```python
from build123d import *

# Parameters (mm, degrees)
SKETCH6_R           = 26
BOSS_EXTRUDE1_DEPTH = 10
CUT_EXTRUDE3_DEPTH  = 39.105117767
CIRPATTERN2_COUNT   = 24
CUT_EXTRUDE4_DEPTH  = 38.897178127
SKETCH9_R           = 5
BOSS_EXTRUDE2_DEPTH = 4


with BuildPart() as part:
    # Sketch6 → Boss-Extrude1 (new body)
    with BuildSketch(Plane.XY):
        Circle(SKETCH6_R)
    extrude(amount=BOSS_EXTRUDE1_DEPTH)

    # Sketch7 → Cut-Extrude3 (cut, through all)
    with BuildSketch(Plane.XY.offset(10)):
        with BuildLine():
            ThreePointArc((-0.990237597, 21.477183929), (-1.515765167, 23.822734617), (-2.811039843, 25.847592828))
            ThreePointArc((-2.811039843, 25.847592828), (0, 26), (2.811039843, 25.847592828))
            ThreePointArc((2.811039843, 25.847592828), (1.515765167, 23.822734617), (0.990237597, 21.477183929))
            ThreePointArc((0.990237597, 21.477183929), (0, 21.5), (-0.990237597, 21.477183929))
        make_face()
    cut_extrude3 = extrude(amount=-CUT_EXTRUDE3_DEPTH, mode=Mode.SUBTRACT)

    # CirPattern2: Cut-Extrude3 ×24 about axis
    cirpattern2_axis = Axis((0, 0, 0), (0, 0, 1))
    for i in range(1, CIRPATTERN2_COUNT):
        add(cut_extrude3.rotate(cirpattern2_axis, i * 360 / CIRPATTERN2_COUNT), mode=Mode.SUBTRACT)

    # Sketch8 → Cut-Extrude4 (cut, through all)
    with BuildSketch(Plane.XY.offset(10)):
        with BuildLine():
            Line((-1.658312395, 2.5), (1.658312395, 2.5))
            ThreePointArc((1.658312395, 2.5), (0, -3), (-1.658312395, 2.5))
        make_face()
    extrude(amount=-CUT_EXTRUDE4_DEPTH, mode=Mode.SUBTRACT)

    # Sketch9 → Boss-Extrude2 (add)
    with BuildSketch(Plane(origin=(0, 0, 0), x_dir=(-1, 0, 0), z_dir=(0, 0, -1))):
        with Locations(Location((0, 0, 0), (0, 0, 180))):
            Circle(SKETCH9_R)
        with BuildLine():
            Line((-1.658312395, 2.5), (1.658312395, 2.5))
            ThreePointArc((1.658312395, 2.5), (0, -3), (-1.658312395, 2.5))
        make_face(mode=Mode.SUBTRACT)
    extrude(amount=BOSS_EXTRUDE2_DEPTH)


solid = part.part
```
Build history of the part. All positions in model axes, mm. A direction names the side the tool comes from. Round coordinates to 2 decimals unless told otherwise and drop trailing zeros. Write each loop counter-clockwise with the first axis right and the second up, starting at its lowest first coordinate (ties: lowest second). Pieces come first, ordered by that corner, then holes.
1) Band-saw the part on B-B, the plane y = -2. List the corners of the cut face in (x, z).
2) Pin check, flat tips, straight feed: pin 1 (2 mm diameter, centred on x = 7, z = 6, fed in from +Y); pin 2 (1 mm diameter, centred on x = -1, z = -1.5, fed in from -Y); pin 3 (2.5 mm diameter, centred on x = 0.5, z = 6.5, fed in from -Y). Stop position of each tip, or through.
3) 3-axis set-ups, long thin cutter, end or side, ignore diameter. For faces 1 (the cylindrical face through (-23.791, -1.503, 5.07)), 2 (the cylindrical face through (22.645, -7.651, 5.07)), 3 (the cylindrical face through (-23.37, 4.706, 5.07)): which of +Z, -Z, +X, -X, +Y, -Y reach the whole face in a straight line?
4) Band-saw the part on D-D, the plane z = -2.5. List the corners of the cut face in (x, y).
5) Drill centre lines: probe 1 along X at (y, z) = (-22, 5.75); probe 2 along X at (y, z) = (20, 8); probe 3 along Y at (x, z) = (0, -1.05). Where is each one in solid material? Low to high.
6) Band-saw the part on C-C, the plane x = 23. List the corners of the cut face in (y, z), and give its area (3 significant figures).
7) Band-saw the part on A-A, the plane x = 0. List the corners of the cut face in (y, z), and give its area (3 significant figures).
8) Mould opens along X. For faces 4 (the cylindrical face through (10.738, -18.626, 5.07)), 5 (the cylindrical face through (-22.59, -7.61, 5.07)), 6 (the cylindrical face through (25.776, -3.402, 4.93)) say: +X half, -X half, draft (parallel to the pull), parting line (faces both ways), or undercut.
Ans:
1. outline: (-24.77, 0) - (-4.58, 0) - (-4.58, -4) - (-2.24, -4) - (-2.24, 10) - (-24.77, 10) - close; (2.24, -4) - (4.58, -4) - (4.58, 0) - (24.77, 0) - (24.77, 10) - (2.24, 10) - close
2. pin 1: stops at y = 23.06
2. pin 2: stops at y = -4.97
2. pin 3: stops at y = -24.33
3. face 1: +Z, -Z, -X
3. face 2: +Z, -Z, +X
3. face 3: +Z, -Z
4. outline: circle Ø10 at (0, 0); hole (-1.66, 2.5) arc R3 ccw (long way) to (1.66, 2.5) - close
5. probe 1: x = -10.65 to -7.2, -4.75 to -1.03, 1.03 to 4.75, 7.2 to 10.65
5. probe 2: x = -16.27 to -13.4, -10.27 to 10.27, 13.4 to 16.27
5. probe 3: y = -5 to -3, 2.5 to 5
6. outline: (-10.62, 0) - (-7.95, 0) - (-7.95, 10) - (-10.62, 10) - close; (-4.74, 0) - (-1.23, 0) - (-1.23, 10) - (-4.74, 10) - close; (1.23, 0) - (4.74, 0) - (4.74, 10) - (1.23, 10) - close; (7.95, 0) - (10.62, 0) - (10.62, 10) - (7.95, 10) - close
6. area: 124 mm2
7. outline: (-21.5, 0) - (-5, 0) - (-5, -4) - (-3, -4) - (-3, 10) - (-21.5, 10) - close; (2.5, -4) - (5, -4) - (5, 0) - (21.5, 0) - (21.5, 10) - (2.5, 10) - close
7. area: 393 mm2
8. face 4: undercut
8. face 5: -X half
8. face 6: +X half
